Build history of the part. All positions in model axes, mm. Face numbers are marked on the shaded views. Round coordinates to 2 decimals unless told otherwise and drop trailing zeros. Write each loop counter-clockwise with the first axis right and the second up, starting at its lowest first coordinate (ties: lowest second). Pieces come first, ordered by that corner, then holes. Notation, with made-up numbers: M 59.25,-8.5 L 107.25,-8.5 A32 cw 107.25,26.5 Z; hole C 68,-32.5 d5. An arc over 180 degrees is marked long. Write item = value, one per line.
from build123d import *

# Parameters (mm, degrees)
SKETCH1_R                           = 9.5
SKETCH1_R_2                         = 1.524
SKETCH1_R_3                         = 2
BOSS_EXTRUDE1_DEPTH                 = 5
CUT_EXTRUDE1_REACH                  = 18.452
CUT_EXTRUDE1_END_RADIUS             = 2
SKETCH3_R                           = 1.524
CUT_EXTRUDE1_DIRECTION_2_REACH      = 18.452
CUT_EXTRUDE1_DIRECTION_2_END_RADIUS = 9.5


with BuildPart() as part:
    # Sketch1 → Boss-Extrude1 (new body)
    with BuildSketch(Plane.XY):
        Circle(SKETCH1_R)
        with Locations((4.490128061, -4.490128061)):
            Circle(SKETCH1_R_2, mode=Mode.SUBTRACT)
        with Locations((-4.490128061, -4.490128061)):
            Circle(SKETCH1_R_2, mode=Mode.SUBTRACT)
        with Locations((-4.490128061, 4.490128061)):
            Circle(SKETCH1_R_2, mode=Mode.SUBTRACT)
        with Locations((4.490128061, 4.490128061)):
            Circle(SKETCH1_R_2, mode=Mode.SUBTRACT)
        Circle(SKETCH1_R_3, mode=Mode.SUBTRACT)
    extrude(amount=BOSS_EXTRUDE1_DEPTH)

    # Cut-Extrude1: up to this cylinder (the profile starts outside it)
    cut_extrude1_end = Plane(origin=(0, 0, 2.5), z_dir=(0, 0, -1)) * Cylinder(CUT_EXTRUDE1_END_RADIUS, 41.904, mode=Mode.PRIVATE)
    # Sketch3 → Cut-Extrude1 (cut, up to the surface)
    with BuildSketch(Plane(origin=(0, 2.966128061, 0), x_dir=(1, 0, 0), z_dir=(0, 1, 0)), mode=Mode.PRIVATE) as cut_extrude1_sk1:
        with Locations(Location((0, -2.5, 0), (0, 0, 180))):
            Circle(SKETCH3_R)
    cut_extrude1_tool1 = extrude(cut_extrude1_sk1.sketch, amount=-CUT_EXTRUDE1_REACH, mode=Mode.PRIVATE) - cut_extrude1_end
    add(cut_extrude1_tool1.solids().sort_by_distance((0, 2.966128, 2.5))[0], mode=Mode.SUBTRACT)

    # Cut-Extrude1 direction 2: up to this cylinder (the profile starts inside it)
    cut_extrude1_direction_2_end = Plane(origin=(0, 0, 2.5), z_dir=(0, 0, -1)) * Cylinder(CUT_EXTRUDE1_DIRECTION_2_END_RADIUS, 56.904, mode=Mode.PRIVATE)
    # Sketch3 → Cut-Extrude1 direction 2 (cut, up to the surface)
    with BuildSketch(Plane(origin=(0, 2.966128061, 0), x_dir=(1, 0, 0), z_dir=(0, 1, 0)), mode=Mode.PRIVATE) as cut_extrude1_direction_2_sk1:
        with Locations(Location((0, -2.5, 0), (0, 0, 180))):
            Circle(SKETCH3_R)
    cut_extrude1_direction_2_tool1 = extrude(cut_extrude1_direction_2_sk1.sketch, amount=CUT_EXTRUDE1_DIRECTION_2_REACH, mode=Mode.PRIVATE) & cut_extrude1_direction_2_end
    add(cut_extrude1_direction_2_tool1.solids().sort_by_distance((0, 2.966128, 2.5))[0], mode=Mode.SUBTRACT)


solid = part.part
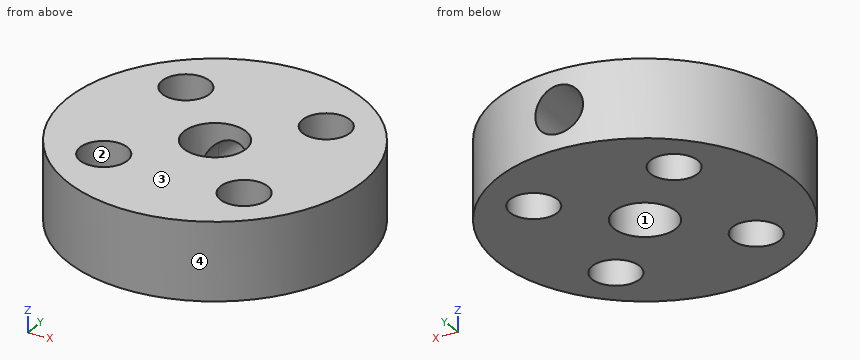
1. Band-saw the part on C-C (z = 2.5). List the corners of the cut face in (x, y), plus the area to 3 significant figures.
Responses:
outline = M -1.52,1.3 L -1.52,9.38 A9.5 ccw long 1.52,9.38 L 1.52,1.3 A2 cw long Z; hole C -4.49,-4.49 d3.05; hole C -4.49,4.49 d3.05; hole C 4.49,-4.49 d3.05; hole C 4.49,4.49 d3.05
area = 218 mm²
2. Mould opens along Y. For the marked faces 1, 2, 3 and 4 say: pulls with the +Y half, pulls with the -Y half, needs draft (parallel to the pull), parting line crosses it, or undercut.
Responses:
face_1 = undercut
face_2 = undercut
face_3 = needs draft
face_4 = parting line crosses it
3. Probe probe 1 along Z at (x, y) = (0, 6.5); probe 2 along X at (y, z) = (5.75, 1.7); probe 3 along Y at (x, z) = (-4.75, 3.5). List the from-to ranges inside material, lowest first.
Responses:
probe_1 = 0 to 0.98, 4.02 to 5
probe_2 = -7.56 to -5.35, -3.63 to -1.3, 1.3 to 3.63, 5.35 to 7.56
probe_3 = -8.23 to -5.99, -2.99 to 2.99, 5.99 to 8.23
4. Band-saw the part on D-D (y = -5.75). List the corners of the cut face in (x, z), plus the area to 3 significant figures.
Responses:
outline = M -7.56,0 L -5.35,0 L -5.35,5 L -7.56,5 Z; M -3.63,0 L 3.63,0 L 3.63,5 L -3.63,5 Z; M 5.35,0 L 7.56,0 L 7.56,5 L 5.35,5 Z
area = 58.5 mm²
5. Flat gauge pins, fed straight in: pin 1 (1.5 mm diameter, centred on x = 1, z = 3.5, fed in from -Y); pin 2 (2.5 mm diameter, centred on x = -4.49, y = -4.49, fed in from +Z); pin 3 (2 mm diameter, centred on x = -7.5, z = 1, fed in from -Y); pin 4 (1.8 mm diameter, centred on x = 0, z = 2.5, fed in from +Y). Where does each tip first touch, or does it go through?
Responses:
pin_1 = -9.5
pin_2 = through
pin_3 = -6.93
pin_4 = -1.79
6. Band-saw the part on B-B (x = 0). List the corners of the cut face in (y, z).
Responses:
outline = M -9.5,0 L -2,0 L -2,5 L -9.5,5 Z; M 2,0 L 9.5,0 L 9.5,0.98 L 2,0.98 Z; M 2,4.02 L 9.5,4.02 L 9.5,5 L 2,5 Z
7. Band-saw the part on A-A (y = 0). List the corners of the cut face in (x, z), plus the area to 3 significant figures.
Responses:
outline = M -9.5,0 L -2,0 L -2,5 L -9.5,5 Z; M 2,0 L 9.5,0 L 9.5,5 L 2,5 Z
area = 75.0 mm²
